Check sheet for the modelled part. Datum: model origin and axes. Units: mm. A direction names the side the tool comes from. Give positions to 0.01 mm unless a question says otherwise; leave off trailing zeros. Order: outer loops, then holes, each group sorted by start corner. A loop starts at its lowest first (then second) coordinate and runs counter-clockwise, first axis right, second up. Notation, with made-up numbers: (78.5, 11.5) -> (84.5, 11.5) arc R32 ccw to (84.5, 42.5) -> close; hole circle Ø2 at (50.25, 48.25). An arc over 180 degrees is marked (long way). One line per question, with ' | ' between items.
```python
from build123d import *

# Parameters (mm, degrees)
SKETCH_1_R          = 2.5
EXTRUDE_1_DEPTH     = 3
SKETCH_2_W          = 3
SKETCH_2_H          = 37
CUT_EXTRUDE_1_DEPTH = 59.579181566
FILLET_1_R          = 1.5


with BuildPart() as part:
    # 草图1 → 凸台-拉伸1 (new body)
    with BuildSketch(Plane.XY):
        Polygon((-18, 19.693473392), (18, 19.693473392), (18, -48.306526608), (33, -48.306526608), (33, 34.693473392), (-33, 34.693473392), (-33, -48.306526608), (-18, -48.306526608), align=None)
        with Locations((0, 28.030377616)):
            Circle(SKETCH_1_R, mode=Mode.SUBTRACT)
        with Locations((25.11473671, -15.469622384)):
            Circle(SKETCH_1_R, mode=Mode.SUBTRACT)
        with Locations((-25.11473671, -15.469622384)):
            Circle(SKETCH_1_R, mode=Mode.SUBTRACT)
    extrude(amount=EXTRUDE_1_DEPTH)

    # 草图2 → 切除-拉伸1 (cut, through all)
    with BuildSketch(Plane.XY.offset(3)):
        with Locations((25.5, 11.693473392)):
            Rectangle(SKETCH_2_W, SKETCH_2_H)
        with Locations((-25.5, 11.693473392)):
            Rectangle(SKETCH_2_W, SKETCH_2_H)
    extrude(amount=-CUT_EXTRUDE_1_DEPTH, mode=Mode.SUBTRACT)

    # 圆角1
    fillet_1_edges = [part.edges().sort_by_distance(p)[0] for p in [
        (27, 30.193473392, 1.5),
        (24, 30.193473392, 1.5),
        (24, -6.806526608, 1.5),
        (27, -6.806526608, 1.5),
        (-24, -6.806526608, 1.5),
        (-27, -6.806526608, 1.5),
        (-24, 30.193473392, 1.5),
        (-27, 30.193473392, 1.5),
    ]]
    fillet(fillet_1_edges, radius=FILLET_1_R - 0.0001)  # a hair under: the kernel refuses the full size


solid = part.part
```
Q1. Access from +Z, -Z, +X, -X, +Y, -Y to the whole of each face (thin tool, end or side, straight path). Record for faces 4 (the face through (18, -14, 1)), 5 (the face through (-26, -48.307, 1)), 6 (the face through (-27, 11, 2)).
Result sheet:
face 4: +Z, -Z, -Y | face 5: +Z, -Z, +X, -X, -Y | face 6: +Z, -Z
Q2. Depth check by flat-ended pin: pin 1 Ø1.5 at (x, y) = (-25, -5.5) entering from -Z; pin 2 Ø8 at (x, y) = (0, 28.03) entering from -Z. Enter the tip coordinate at first touch or a pass-through.
Result sheet:
pin 1: passes through | pin 2: stops at z = 0
Q3. Section check A-A (y = -10). Enter the section's corners in (x, z).
Result sheet:
outline: (-33, 0) -> (-18, 0) -> (-18, 3) -> (-33, 3) -> close; (18, 0) -> (33, 0) -> (33, 3) -> (18, 3) -> close
Q4. Section check D-D (z = 1.9). Count the separate pieces of the cut face and the enclosed holes in it, and give its area (3 significant figures).
Result sheet:
separate pieces: 1 | enclosed holes: 5 | area: 2,750 mm2
Q5. Mould release check, pull along X, two halves, no side actions. Record for faces 1 (the face through (33, -7, 1)), 2 (the face through (0, 19.693, 1)), 3 (the face through (0, 21, 3)): pulls with the +X half, pulls with the -X half, needs draft (parallel to the pull), parting line crosses it, or undercut.
Result sheet:
face 1: pulls with the +X half | face 2: undercut | face 3: needs draft
Q6. Thickness scan on line 1 (X direction, y = 9.5, z = 2.2); line 2 (X direction, y = 20, z = 2.05); line 3 (X direction, y = -12, z = 1.7). Record the ranges inside material, lowest first.
Result sheet:
line 1: x = -33 to -27, -24 to -18, 18 to 24, 27 to 33 | line 2: x = -33 to -27, -24 to 24, 27 to 33 | line 3: x = -33 to -18, 18 to 33
Q7. Section check C-C (x = 0). Enter the section's corners in (y, z).
Result sheet:
outline: (19.69, 0) -> (25.53, 0) -> (25.53, 3) -> (19.69, 3) -> close; (30.53, 0) -> (34.69, 0) -> (34.69, 3) -> (30.53, 3) -> close
Q8. Section check B-B (y = 6.5). Enter the section's corners in (x, z), and give its area (3 significant figures).
Result sheet:
outline: (-33, 0) -> (-27, 0) -> (-27, 3) -> (-33, 3) -> close; (-24, 0) -> (-18, 0) -> (-18, 3) -> (-24, 3) -> close; (18, 0) -> (24, 0) -> (24, 3) -> (18, 3) -> close; (27, 0) -> (33, 0) -> (33, 3) -> (27, 3) -> close | area: 72.0 mm2
